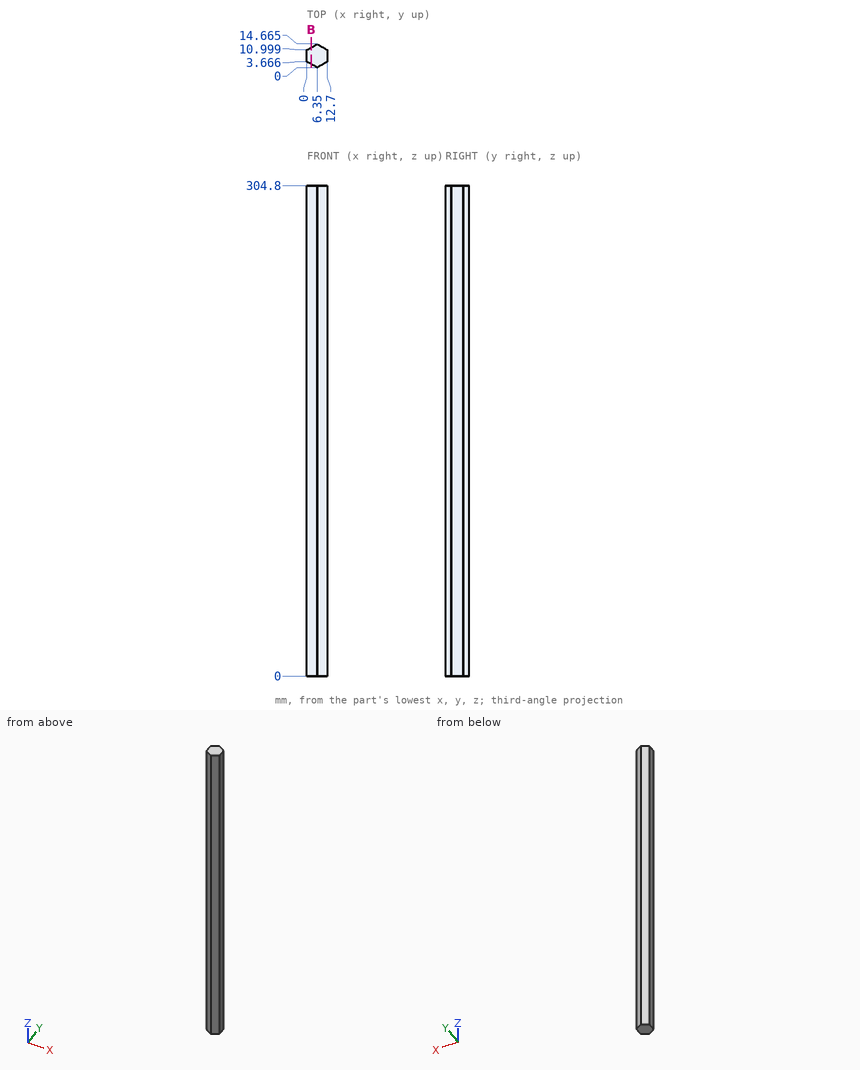
Print and shaded views of the part. All mm, measured from the part's lowest x, y and z. Give positions to 0.01 mm unless a question says otherwise; leave off trailing zeros. Write each loop counter-clockwise with the first axis right and the second up, starting at its lowest first coordinate (ties: lowest second). Pieces come first, ordered by that corner, then holes. Notation, with made-up numbers: M 84,22.25 L 98,22.25 A22 cw 98,51.25 Z; hole C 11.25,13 d4. An arc over 180 degrees is marked long. Use a Markdown table: item, result.
1) Pin check, flat tips, straight feed: pin 1 (4 mm diameter, centred on x = 4, z = 78, fed in from -Y); pin 2 (5 mm diameter, centred on x = 9, y = 4.5, fed in from -Z); pin 3 (1.5 mm diameter, centred on y = 12, z = 112.5, fed in from -X) (1 decimal); pin 4 (1 mm diameter, centred on y = 12.5, z = 33.5, fed in from -X) (1 decimal). Stop position of each tip, or through.
Responses:
| item | result |
|---|---|
| pin 1 | stops at y = 0.2 |
| pin 2 | stops at z = 0 |
| pin 3 | stops at x = 0.4 |
| pin 4 | stops at x = 1.7 |
2) Drill centre lines: line 1 (Y direction, x = 6.5, z = 162.5) (1 decimal); line 2 (Y direction, x = 11.5, z = 281) (1 decimal); line 3 (X direction, y = 14.25, z = 194) (1 decimal). Where is each one in solid material? Low to high. Write a range as from..to.
Responses:
| item | result |
|---|---|
| line 1 | y = 0.1..14.6 |
| line 2 | y = 3..11.7 |
| line 3 | x = 5.6..7.1 |
3) Cut at B-B (x = 2.5). List the corners of the cut face in (y, z).
Responses:
| item | result |
|---|---|
| outline | M 2.22,0 L 12.44,0 L 12.44,304.8 L 2.22,304.8 Z |
